```python
from build123d import *

# Parameters (mm, degrees)
F2_DEPTH = 25
F0_R     = 51.030989
F3_DEPTH = 92.821598


with BuildPart() as f2:
    # F1 (on Front) → F2 (new body)
    with BuildSketch(Plane.XZ):
        with BuildLine():
            ThreePointArc((74.871618, -4.386429), (48.102518, 13.643599), (61.418848, 43.043293))
            ThreePointArc((61.418848, 43.043293), (-72.153777, -20.465398), (74.871618, -4.386429))
        make_face()
    extrude(amount=F2_DEPTH)

    # F0 (on Front) → F3 (join)
    with BuildSketch(Plane.XZ):
        Circle(F0_R)
    extrude(amount=F3_DEPTH)


solid = f2.part
```
Build history of the part. All positions in model axes, mm. A direction names the side the tool comes from. Round coordinates to 2 decimals unless told otherwise and drop trailing zeros. Loops run counter-clockwise (first coordinate to the right, second up) from the corner with the lowest first, then second, coordinate; pieces in that order, holes last.
Item 1: Drill centre lines: line 1 along Y through (x, z) = (-26.5, -50.5); line 2 along X through (y, z) = (-64, 0.5); line 3 along Z through (x, y) = (1.5, -66). Where is each one in solid material? Low to high.
Item 2: Two-plate mould, pull along Z, no slides. Class faces 1 (the face through (-1, 0, 1)), 2 (the face through (-72.9, -12.32, -17.62)), 3 (the face through (60.911, -12.325, -1.864)): released by +Z, released by -Z, zero draft, split by the parting line, or undercut.
Item 3: Saw through at C-C (y = -32). List the corners of the cut face in (x, z), then the cut area to 3 significant figures.
Item 4: Saw through at A-A (x = 0). List the corners of the cut face in (y, z), then the cut area to 3 significant figures.
Item 5: Which spindle directions (+Z, -Z, +X, -X, +Y, -Y) get a long thin tool onto all of the face, cutting with end or side? Do faces 4 (the face through (50.65, -12.32, 33.22)), 5 (the face through (48.674, -56.075, 15.328)), 6 (the face through (-1, -92.822, 1)). Say none if no direction does.
Item 6: Saw through at B-B (z = 34). List the corners of the cut face in (x, y).
Item 7: Pin check, flat tips, straight feed: P1, Ø1.5, axis at y = -34, z = 40.5, coming from the +X side; P2, Ø8, axis at x = -29.5, y = -19, coming from the -Z side; P3, Ø4, axis at x = 46, y = -20, coming from the +Z side. Stop position of each tip, or through.
Item 8: Saw through at D-D (x = -53.5). List the corners of the cut face in (y, z), then the cut area to 3 significant figures.
Worked answers:
1. line 1: y = -25 to 0
1. line 2: x = -51.03 to 51.03
1. line 3: z = -51.01 to 51.01
2. face 1: zero draft
2. face 2: split by the parting line
2. face 3: undercut
3. outline: circle Ø102.06 at (0, 0)
3. area: 8,180 mm2
4. outline: (-92.82, -51.03) - (-25, -51.03) - (-25, -75) - (0, -75) - (0, 75) - (-25, 75) - (-25, 51.03) - (-92.82, 51.03) - close
4. area: 10,700 mm2
5. face 4: +X, +Y, -Y
5. face 5: -Y
5. face 6: +Z, -Z, +X, -X, -Y
6. outline: (-66.85, -25) - (-38.05, -25) - (-38.05, -92.82) - (38.05, -92.82) - (38.05, -25) - (51.13, -25) - (51.13, 0) - (-66.85, 0) - close
7. P1: stops at x = 32
7. P2: stops at z = -70.53
7. P3: stops at z = 60.74
8. outline: (-25, -52.56) - (0, -52.56) - (0, 52.56) - (-25, 52.56) - close
8. area: 2,630 mm2
